The model under review builds one solid part; all positions refer to its coordinate system, in mm. A direction names the side the tool comes from. Coordinates: 2 decimals unless noted, no trailing zeros. Order: outer loops, then holes, each group sorted by start corner. A loop starts at its lowest first (then second) coordinate and runs counter-clockwise, first axis right, second up. Notation, with made-up numbers: (-4.75, -35.5) -> (37.25, -35.5) arc R22 ccw to (37.25, -23.5) -> close; hole circle Ø3 at (-37, 77.5). An arc over 180 degrees is marked (long way). Use CSV: the item, a comma, the result in double quotes. Start each with the question number.
Autodesk Fusion 360 part; units mm, degrees
sketch "草图1" plane through (0, 0, 0) normal (0, 1, 0) x (1, 0, 0)
  circle A0 centre (0, 0) radius 46.5
  circle A1 centre (0, 0) radius 33
  circle A2 centre (0, 0) radius 48.5
  circle A3 centre (0, 0) radius 35
  dimension "d1" = 93
  dimension "d2" = 66
  dimension "d3" = 97
  dimension "d4" = 70
extrude "拉伸3" add sketch "草图1" along normal blind 60 draft 12.7 contours A3
extrude "拉伸4" cut sketch "草图1" along normal blind 60 draft 12.7 contours A1
extrude "拉伸5" add sketch "草图1" against normal blind 60 contours A3
sketch "草图2" plane through (0, -60, 0) normal (0, -1, 0) x (1, 0, 0)
  circle A0 centre (0, 0) radius 33
  circle A1 centre (0, 0) radius 35
extrude "拉伸6" add sketch "草图2" along normal blind 60 draft 12.7
extrude "拉伸7" cut sketch "草图2" along normal blind 60 draft 12.7 contours A0
sketch "草图3" plane through (0, -120, 0) normal (0, -1, 0) x (1, 0, 0)
  circle A0 centre (0, 0) radius 46.5216
  circle A1 centre (0, 0) radius 48.5216
extrude "拉伸8" add sketch "草图3" against normal blind 2 draft 12.7 contours A0
Q1. Add section B-B, the plane y = -19. State the section outline as (x, z) points, then the cut area to 3 significant figures.
Q2. To check wall thickness, follow probe 1 along X at (y, z) = (-27, 0); probe 2 along X at (y, z) = (-30.5, -22.5). State the ranges of each line that lie inside material, in increasing order.
Q3. Add section D-D, the plane x = 0. State the section outline as (y, z) points, then the cut area to 3 significant figures.
Q4. Add section A-A, the plane z = 0. State the section outline as (x, y) points, then the cut area to 3 significant figures.
Q5. Clearance check with flat-ended pins moving along their axes: pin 1 Ø1 at (x, z) = (8.5, 25.5) entering from +Y; pin 2 Ø1 at (x, y) = (-29, 32) entering from -Z; pin 3 Ø6 at (y, z) = (-66, 29.5) entering from +X. State where each tip first meets the part, or that it passes through.
Q6. Draft analysis for pull direction Y (two halves, no side actions). For faces 1 (the conical face through (38.49, 23.75, -12.12)), 2 (the conical face through (-8.31, 23.75, 37.44)), 3 (the flat face through (-1, -120, 1)), state which applies: +Y half, -Y half, draft (parallel to the pull), parting line (faces both ways), or undercut.
Q7. For faces 4 (the cylindrical face through (-28, -30, 21)), 5 (the cylindrical face through (30.5, -29.6, 12.6)), list the 3-axis set-ups (+Z, -Z, +X, -X, +Y, -Y) from which the entire face can be reached by the end or side of a thin tool; tool diameter is ignored.
Q8. Add section C-C, the plane x = 41. State how many separate pieces and enclosed holes the cut face has, then the cut area to 3 significant figures.
Answer block:
1,outline,"circle Ø70 at (0, 0); hole circle Ø66 at (0, 0)"
1,area,"427 mm²"
2,probe 1,"x = -35 to -33, 33 to 35"
2,probe 2,"x = -26.81 to -24.14, 24.14 to 26.81"
3,outline,"(-120, -48.52) -> (-60, -35) -> (0, -35) -> (60, -48.52) -> (60, -46.52) -> (0, -33) -> (-60, -33) -> (-118, -46.07) -> (-118, 46.07) -> (-60, 33) -> (0, 33) -> (60, 46.52) -> (60, 48.52) -> (0, 35) -> (-60, 35) -> (-120, 48.52) -> close"
3,area,"905 mm²"
4,outline,"(-48.52, -120) -> (48.52, -120) -> (35, -60) -> (35, 0) -> (48.52, 60) -> (46.52, 60) -> (33, 0) -> (33, -60) -> (46.07, -118) -> (-46.07, -118) -> (-33, -60) -> (-33, 0) -> (-46.52, 60) -> (-48.52, 60) -> (-35, 0) -> (-35, -60) -> close"
4,area,"905 mm²"
5,pin 1,"stops at y = -118"
5,pin 2,"stops at z = -31.16"
5,pin 3,"stops at x = 25.03"
6,face 1,"undercut"
6,face 2,"+Y half"
6,face 3,"-Y half"
7,face 4,"none"
7,face 5,"+Y"
8,separate pieces,"2"
8,enclosed holes,"1"
8,area,"938 mm²"
